```python
from build123d import *

# Parameters (mm, degrees)
SKETCH1_W           = 160
SKETCH1_H           = 25
BOSS_EXTRUDE1_DEPTH = 5
SKETCH2_R           = 1.25
SKETCH2_R_2         = 1.24
CUT_EXTRUDE1_DEPTH  = 10
SKETCH5_W           = 1.5
SKETCH5_H           = 2
CUT_EXTRUDE4_DEPTH  = 163.01851746
SKETCH6_R           = 1.25
CUT_EXTRUDE5_DEPTH  = 10
SKETCH7_R           = 1.25
CUT_EXTRUDE6_DEPTH  = 10
CUT_EXTRUDE7_START  = -10
SKETCH8_R           = 1.25
CUT_EXTRUDE7_DEPTH  = 10


with BuildPart() as part:
    # Sketch1 → Boss-Extrude1 (new body)
    with BuildSketch(Plane.XY):
        with Locations((80, 12.5)):
            Rectangle(SKETCH1_W, SKETCH1_H)
    extrude(amount=BOSS_EXTRUDE1_DEPTH)

    # Sketch2 → Cut-Extrude1 (cut)
    with BuildSketch(Plane.XZ):
        with Locations(Location((40, 2.5, 0), (0, 0, 270))):
            Circle(SKETCH2_R)
        with Locations(Location((120, 2.5, 0), (0, 0, 270))):
            Circle(SKETCH2_R_2)
    extrude(amount=-CUT_EXTRUDE1_DEPTH, mode=Mode.SUBTRACT)

    # Sketch5 → Cut-Extrude4 (cut, through all)
    with BuildSketch(Plane.ZY):
        with Locations((0.75, 20)):
            Rectangle(SKETCH5_W, SKETCH5_H)
    extrude(amount=-CUT_EXTRUDE4_DEPTH, mode=Mode.SUBTRACT)

    # Sketch6 → Cut-Extrude5 (cut)
    with BuildSketch(Plane.XY.offset(5)):
        with Locations((40, 12.5)):
            Circle(SKETCH6_R)
        with Locations((120, 12.5)):
            Circle(SKETCH6_R)
    extrude(amount=-CUT_EXTRUDE5_DEPTH, mode=Mode.SUBTRACT)

    # Sketch7 → Cut-Extrude6 (cut)
    with BuildSketch(Plane.ZY):
        with Locations((2.5, 5)):
            Circle(SKETCH7_R)
        with Locations((2.5, 15)):
            Circle(SKETCH7_R)
    extrude(amount=-CUT_EXTRUDE6_DEPTH, mode=Mode.SUBTRACT)

    # Sketch8 → Cut-Extrude7 (cut)
    with BuildSketch(Plane(origin=(160, 0, 0), x_dir=(0, 0, -1), z_dir=(1, 0, 0)).offset(CUT_EXTRUDE7_START)):
        with Locations(Location((-2.5, 5, 0), (0, 0, 180))):
            Circle(SKETCH8_R)
        with Locations(Location((-2.5, 15, 0), (0, 0, 180))):
            Circle(SKETCH8_R)
    extrude(amount=CUT_EXTRUDE7_DEPTH, mode=Mode.SUBTRACT)


solid = part.part
```
CAD build for the part. Positions are in the model's coordinates, mm. A direction names the side the tool comes from. Round coordinates to 2 decimals unless told otherwise and drop trailing zeros. Write each loop counter-clockwise with the first axis right and the second up, starting at its lowest first coordinate (ties: lowest second). Pieces come first, ordered by that corner, then holes.
Item 1: Drop flat-ended pins along their axis: pin 1 Ø1.5 at (y, z) = (5, 2.5) entering from +X; pin 2 Ø2 at (y, z) = (15, 2.5) entering from -X; pin 3 Ø2 at (x, z) = (120, 2.5) entering from -Y. Give the stop position or say it passes through.
Filled in:
pin 1: stops at x = 150
pin 2: stops at x = 10
pin 3: stops at y = 10
Item 2: Tool access for faces 4 (the flat face through (120, 10, 3)), 5 (the flat face through (10, 5, 2)), 6 (the flat face through (79, 25, 2)), 7 (the flat face through (150, 15, 2)): list every direction of +Z, -Z, +X, -X, +Y, -Y with a clear straight run to the whole face (end or side of a thin tool).
Filled in:
face 4: -Y
face 5: -X
face 6: +Z, -Z, +X, -X, +Y
face 7: +X
Item 3: Band-saw the part on A-A on z = 2.5. Give the number of separate pieces and of enclosed holes in the cut face, then the cut area to 3 significant figures.
Filled in:
separate pieces: 1
enclosed holes: 2
area: 3,840 mm2
Item 4: Mould opens along X. For faces 1 (the cylindrical face through (4.93, 16.054, 3.172)), 2 (the cylindrical face through (121.23, 4.93, 2.66)), 3 (the flat face through (150, 5, 2)) say: released by +X, released by -X, zero draft, split by the parting line, or undercut.
Filled in:
face 1: zero draft
face 2: undercut
face 3: released by +X
Item 5: Drill centre lines: L1, parallel to X at y = 2.5, z = 2.5; L2, parallel to Y at x = 155, z = 2.5; L3, parallel to Z at x = 155.75, y = 15. Where is each one in solid material? Low to high.
Filled in:
L1: x = 0 to 38.75, 41.25 to 118.76, 121.24 to 160
L2: y = 0 to 3.75, 6.25 to 13.75, 16.25 to 25
L3: z = 0 to 1.25, 3.75 to 5
Item 6: Band-saw the part on B-B on x = 97.5. Write the cut outline in (y, z), then the cut area to 3 significant figures.
Filled in:
outline: (0, 0) - (19, 0) - (19, 1.5) - (21, 1.5) - (21, 0) - (25, 0) - (25, 5) - (0, 5) - close
area: 122 mm2
